Read the model definition and answer for the solid it produces. Units are mm, in the model's axes. A direction names the side the tool comes from. Coordinates: 2 decimals unless noted, no trailing zeros. Loops run counter-clockwise (first coordinate to the right, second up) from the corner with the lowest first, then second, coordinate; pieces in that order, holes last. Notation, with made-up numbers: M 70.25,-5.5 L 129.25,-5.5 A8 ccw 129.25,-1.5 Z; hole C -12.5,-30.5 d1. An arc over 180 degrees is marked long. One line per item, written item: value. Start each with the question number.
1. A flat-ended cylindrical pin translates along its axis: pin 1 (8 mm diameter, centred on x = -46, z = -2.5, fed in from +Y). Find the tip coordinate at first contact, or state that the pin passes through.
2. Determine the mould class of faces 1 (the face through (-3, 18, -250)), 2 (the face through (250, 18, 3)), 3 (the face through (247, 20, 3)) for opening direction X: +X half, -X half, draft (parallel to the pull), parting line (faces both ways), or undercut.
3. The part is cut by section A-A (y = 12). Write down the section's boundary in (x, z).
4. The part is cut by section C-C (z = 46.5). Write down the section's boundary in (x, y).
5. For faces 4 (the face through (236, 34, 238)), 5 (the face through (-250, 18, 3)), determine the directions among +Z, -Z, +X, -X, +Y, -Y from which every point of the face is accessible in a straight line to the end or side of a thin tool.
6. The part is cut by section B-B (x = 141). Write down the section's boundary in (y, z), then the cut area to 3 significant figures.
7. Consider probe 1 along Z at (x, y) = (240, 35.1); probe 2 along X at (y, z) = (0.8, 113); probe 3 along X at (y, z) = (2, 240). Determine where each line is inside the solid, lowest interval first.
```python
from build123d import *

# Parameters (mm, degrees)
SKETCH1_W           = 500
SKETCH1_H           = 500
BOSS_EXTRUDE1_DEPTH = 37
SHELL1_T            = -3
SKETCH3_R           = 2.5
CUT_EXTRUDE1_DEPTH  = 37
SKETCH4_W           = 17
SKETCH4_H           = 17
BOSS_EXTRUDE2_DEPTH = 3
SKETCH5_R           = 2.5
CUT_EXTRUDE2_DEPTH  = 3


with BuildPart() as part:
    # Sketch1 → Boss-Extrude1 (new body)
    with BuildSketch(Plane(origin=(0, 0, 0), x_dir=(1, 0, 0), z_dir=(0, 1, 0))):
        Rectangle(SKETCH1_W, SKETCH1_H)
    extrude(amount=BOSS_EXTRUDE1_DEPTH)

    # Shell1
    shell1_openings = [part.faces().sort_by_distance(p)[0] for p in [
        (0, 37, 0),
    ]]
    offset(amount=SHELL1_T, openings=shell1_openings, kind=Kind.INTERSECTION)

    # Sketch3 → Cut-Extrude1 (cut)
    with BuildSketch(Plane(origin=(0, 37, 0), x_dir=(1, 0, 0), z_dir=(0, 1, 0))):
        with Locations(Location((113, -240, 0), (0, 0, 270))):
            Circle(SKETCH3_R)
        with Locations(Location((-113, -240, 0), (0, 0, 270))):
            Circle(SKETCH3_R)
        with Locations(Location((240, 113, 0), (0, 0, 270))):
            Circle(SKETCH3_R)
        with Locations(Location((240, -113, 0), (0, 0, 270))):
            Circle(SKETCH3_R)
        with Locations(Location((-240, -113, 0), (0, 0, 270))):
            Circle(SKETCH3_R)
        with Locations(Location((-240, 113, 0), (0, 0, 270))):
            Circle(SKETCH3_R)
        with Locations(Location((-113, 240, 0), (0, 0, 270))):
            Circle(SKETCH3_R)
        with Locations(Location((113, 240, 0), (0, 0, 270))):
            Circle(SKETCH3_R)
    extrude(amount=-CUT_EXTRUDE1_DEPTH, mode=Mode.SUBTRACT)

    # Sketch4 → Boss-Extrude2 (add)
    with BuildSketch(Plane(origin=(0, 37, 0), x_dir=(1, 0, 0), z_dir=(0, 1, 0))):
        with Locations((-238.5, 238.5)):
            Rectangle(SKETCH4_W, SKETCH4_H)
        with Locations((238.5, 238.5)):
            Rectangle(SKETCH4_W, SKETCH4_H)
        with Locations((238.5, -238.5)):
            Rectangle(SKETCH4_W, SKETCH4_H)
        with Locations((-238.5, -238.5)):
            Rectangle(SKETCH4_W, SKETCH4_H)
    extrude(amount=-BOSS_EXTRUDE2_DEPTH)

    # Sketch5 → Cut-Extrude2 (cut)
    with BuildSketch(Plane(origin=(0, 37, 0), x_dir=(1, 0, 0), z_dir=(0, 1, 0))):
        with Locations(Location((-240, 240, 0), (0, 0, 270))):
            Circle(SKETCH5_R)
        with Locations(Location((240, 240, 0), (0, 0, 90))):
            Circle(SKETCH5_R)
        with Locations(Location((240, -240, 0), (0, 0, 270))):
            Circle(SKETCH5_R)
        with Locations(Location((-240, -240, 0), (0, 0, 90))):
            Circle(SKETCH5_R)
    extrude(amount=-CUT_EXTRUDE2_DEPTH, mode=Mode.SUBTRACT)


solid = part.part
```
Answer block:
1. pin 1: stops at y = 3
2. face 1: draft
2. face 2: +X half
2. face 3: undercut
3. outline: M -250,-250 L 250,-250 L 250,250 L -250,250 Z; hole M -247,-247 L 247,-247 L 247,247 L -247,247 Z
4. outline: M -250,0 L 250,0 L 250,37 L 247,37 L 247,3 L -247,3 L -247,37 L -250,37 Z
5. face 4: none
5. face 5: +Z, -Z, -X, +Y, -Y
6. outline: M 0,-250 L 37,-250 L 37,-247 L 3,-247 L 3,247 L 37,247 L 37,250 L 0,250 Z
6. area: 1,700 mm2
7. probe 1: z = -250 to -242.5, -237.5 to -230, 230 to 237.5, 242.5 to 250
7. probe 2: x = -250 to -242.5, -237.5 to 237.5, 242.5 to 250
7. probe 3: x = -250 to -115.5, -110.5 to 110.5, 115.5 to 250
